Autodesk Inventor part; units mm, degrees
ref_plane "Work Plane3" through (0, 0, 178) normal (0, 0, 1) x (1, 0, 0)
ref_plane "Work Plane2" through (0, 0, 4) normal (0, 0, 1) x (1, 0, 0)
ref_plane "YZ Plane" through (0, 0, 0) normal (1, 0, 0) x (0, 1, 0)
ref_plane "Work Plane1" through (0, 0, 4) normal (0, 0, 1) x (1, 0, 0)
sketch "Sketch2" plane through (0, 0, 4) normal (0, 0, 1) x (1, 0, 0)
  circle A0 centre (0, 0) radius 300
  circle A1 centre (0, 0) radius 25
  circle A2 centre (0, 0) radius 15
  dimension "d3" = 50
  dimension "d4" = 30
extrude "Extrusion2" add sketch "Sketch2" along normal blind 50 contours A1 | A2
extrude "Extrusion3" add sketch "Sketch2" along normal blind 174 contours A2
ref_plane "Work Plane3" through (0, 0, 178) normal (0, 0, 1) x (1, 0, 0)
sketch "Sketch3" plane through (0, 0, 178) normal (0, 0, 1) x (1, 0, 0)
  circle A0 centre (0, 0) radius 15
  circle A1 centre (0, 0) radius 9
  dimension "d9" = 18
extrude "Extrusion4" add sketch "Sketch3" along normal blind 20 contours A1
ref_plane "Work Plane2" through (0, 0, 4) normal (0, 0, 1) x (1, 0, 0)
sketch "Sketch4" plane through (0, 0, 4) normal (0, 0, 1) x (1, 0, 0)
  circle A0 centre (0, 0) radius 25
  circle A1 centre (0, 0) radius 300
  line L0 (0, 0) -> (0, 300)
  line L1 (0, 0) -> (0, -300)
  line L2 (0, 0) -> (300, 0)
fillet "Fillet2" radius 9 1 edges at (-9, 0, 198)
properties part number "Lilin"
Design review of the part built by this model. Coordinates are the model's own, in mm. A direction names the side the tool comes from. Coordinates: 2 decimals unless noted, no trailing zeros. Order: outer loops, then holes, each group sorted by start corner. A loop starts at its lowest first (then second) coordinate and runs counter-clockwise, first axis right, second up. Notation, with made-up numbers: (61, 87.25) -> (103, 87.25) arc R23 cw to (103, 114.25) -> close; hole circle Ø7 at (0, -6). An arc over 180 degrees is marked (long way). Use one line per item in the form item = value. Start each with the question number.
(1) For faces 1 (the cylindrical face through (-1.172, -8.923, 183.423)), 2 (the flat face through (0, 0, 4)), list the 3-axis set-ups (+Z, -Z, +X, -X, +Y, -Y) from which the entire face can be reached by the end or side of a thin tool; tool diameter is ignored.
(2) Insertion check: pin 1 (2 mm diameter, centred on y = 9.5, z = 118, fed in from +X); pin 2 (1.5 mm diameter, centred on x = 16, y = 0, fed in from +Z); pin 3 (4 mm diameter, centred on x = 10.5, y = 5, fed in from +Z). Each pin has a flat end and moves straight along its axis. Give the tip position at first contact, or say it passes through.
(3) For probe 1 along X at (y, z) = (1, 59.5); probe 2 along Z at (x, y) = (17.5, 10); probe 3 along Z at (x, y) = (-12.5, 1), list the stretches that pass through material, from the lowest coordinate up.
(4) Add section D-D on y = 11. State the section outline as (x, z) points.
(5) Add section C-C on z = 120. State the section outline as (x, y) points.
(6) Add section A-A on y = 0. State the section outline as (x, z) points, plus the area to 3 significant figures.
Answer block:
q1.face_1 = +Z
q1.face_2 = -Z, +X, -X, +Y, -Y
q2.pin_1 = 12.36
q2.pin_2 = 54
q2.pin_3 = 178
q3.probe_1 = -14.97 to 14.97
q3.probe_2 = 4 to 54
q3.probe_3 = 4 to 178
q4.outline = (-22.45, 4) -> (22.45, 4) -> (22.45, 54) -> (10.2, 54) -> (10.2, 178) -> (-10.2, 178) -> (-10.2, 54) -> (-22.45, 54) -> close
q5.outline = circle Ø30 at (0, 0)
q6.outline = (-25, 4) -> (25, 4) -> (25, 54) -> (15, 54) -> (15, 178) -> (9, 178) -> (9, 189) arc R9 ccw to (-9, 189) -> (-9, 178) -> (-15, 178) -> (-15, 54) -> (-25, 54) -> close
q6.area = 6,550 mm²
